Could you check a few things on this model? Use its own coordinates, in mm. Round coordinates to 2 decimals unless told otherwise and drop trailing zeros. Write each loop counter-clockwise with the first axis right and the second up, starting at its lowest first coordinate (ties: lowest second). Pieces come first, ordered by that corner, then holes. Notation, with made-up numbers: (69, 60) - (117, 60) arc R24 cw to (117, 78) - close; hole circle Ø4 at (29.25, 13). An arc over 180 degrees is marked (long way). Write each question's results on one line, items separated by ' | '. Start each with the question number.
(1) Imagine slicing it at B-B on y = 3. Write out the boundary of the cut face in (x, z), then the cut area to 3 significant figures.
(2) Imagine slicing it at A-A on x = -24.5. Write out the boundary of the cut face in (y, z).
(3) Please list where these lines run through material, in increasing order: line 1 (Y direction, x = 8, z = 0.15); line 2 (Y direction, x = 22.5, z = 0.2); line 3 (X direction, y = 2, z = 0.3). Write a range as [from, to].
(4) Imagine slicing it at D-D on x = 33.5. Write out the boundary of the cut face in (y, z), then the cut area to 3 significant figures.
(5) Imagine slicing it at C-C on z = 0.2. Write out the boundary of the cut face in (x, y), then the cut area to 3 significant figures.
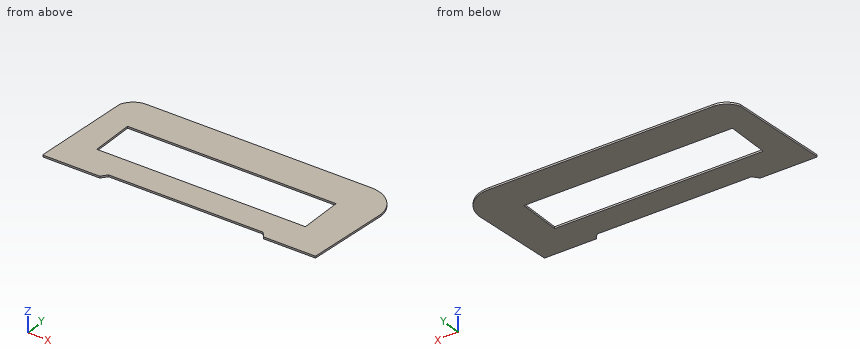
```python
from build123d import *

# Parameters (mm, degrees)
F0_W     = 57.3139749467
F0_H     = 12.0063517243
F1_DEPTH = 0.508


# Not quite as in the source:
# - ends of sketch curves that miss each other by under 0.0002 mm in the source are joined


with BuildPart() as f1:
    # F0 (on Top) → F1 (new body)
    with BuildSketch(Plane.XY):
        with BuildLine():
            Line((-36.7499960837, 12.0419642886), (-38.4861308, -15.2827228))
            ThreePointArc((-38.4861308, -15.2827228), (-38.4148753009, -15.4677583266), (-38.2323086, -15.5451301886))
            Line((-38.2323086, -15.5451301886), (-22.7499926, -15.545054))
            Line((-22.7499926, -15.545054), (-21.4799926, -13.9580366))
            Line((-21.4799926, -13.9580366), (20.9799936, -13.9580366))
            Line((20.9799936, -13.9580366), (22.2499936, -15.545054))
            Line((22.2499936, -15.545054), (36.2593128, -15.545054))
            ThreePointArc((36.2593128, -15.545054), (36.4352434048, -15.4742599559), (36.5131044113, -15.3013407897))
            Line((36.5131044113, -15.3013407897), (38.2500089611, 7.7244699848))
            ThreePointArc((38.2500089611, 7.7244699848), (35.5514966121, 13.3615420014), (29.6945050156, 15.5419546358))
            Line((29.6945050156, 15.5419546358), (-31.9416938, 15.5419806))
            ThreePointArc((-31.9416938, 15.5419806), (-34.897631264, 14.5500112443), (-36.7499960837, 12.0419642886))
        make_face()
        with Locations((-1.2608356774, -0.5606063642)):
            Rectangle(F0_W, F0_H, mode=Mode.SUBTRACT)
    extrude(amount=F1_DEPTH)


solid = f1.part
```
Response:
1) outline: (-37.32, 0) - (-29.92, 0) - (-29.92, 0.51) - (-37.32, 0.51) - close; (27.4, 0) - (37.89, 0) - (37.89, 0.51) - (27.4, 0.51) - close | area: 9.10 mm²
2) outline: (-15.55, 0) - (-6.56, 0) - (-6.56, 0.51) - (-15.55, 0.51) - close; (5.44, 0) - (15.54, 0) - (15.54, 0.51) - (5.44, 0.51) - close
3) line 1: [-13.96, -6.56], [5.44, 15.54] | line 2: [-15.55, -6.56], [5.44, 15.54] | line 3: [-37.39, -29.92], [27.4, 37.82]
4) outline: (-15.55, 0) - (14.74, 0) - (14.74, 0.51) - (-15.55, 0.51) - close | area: 15.4 mm²
5) outline: (-38.49, -15.28) arc R0.25 ccw to (-38.23, -15.55) - (-22.75, -15.55) - (-21.48, -13.96) - (20.98, -13.96) - (22.25, -15.55) - (36.26, -15.55) arc R0.25 ccw to (36.51, -15.3) - (38.25, 7.72) arc R8.34 ccw to (29.69, 15.54) - (-31.94, 15.54) arc R5.18 ccw to (-36.75, 12.04) - close; hole (-29.92, -6.56) - (27.4, -6.56) - (27.4, 5.44) - (-29.92, 5.44) - close | area: 1,560 mm²
